from build123d import *

# Parameters (mm, degrees)
BOSS_EXTRUDE1_DEPTH = 12.7
CUT_EXTRUDE1_DEPTH  = 6.35
CUT_EXTRUDE2_DEPTH  = 233.052537155
SKETCH5_R           = 3.675
BOSS_EXTRUDE2_DEPTH = 12.7


with BuildPart() as part:
    # Sketch1 → Boss-Extrude1 (new, symmetric)
    with BuildSketch(Plane.XY):
        with BuildLine():
            Line((0, 163.1), (0, 125))
            ThreePointArc((0, 125), (88.388347648, 88.388347648), (125, 0))
            Line((125, 0), (163.1, 0))
            ThreePointArc((163.1, 0), (115.329116012, 115.329116012), (0, 163.1))
        make_face()
    extrude(amount=BOSS_EXTRUDE1_DEPTH, both=True)

    # Sketch3 → Cut-Extrude1 (cut, symmetric)
    with BuildSketch(Plane.XY):
        with BuildLine():
            Line((25.4, 161.110055552), (19.466584917, 123.474904623))
            ThreePointArc((19.466584917, 123.474904623), (88.388347648, 88.388347648), (123.474904623, 19.466584917))
            Line((123.474904623, 19.466584917), (161.110055552, 25.4))
            ThreePointArc((161.110055552, 25.4), (115.329116012, 115.329116012), (25.4, 161.110055552))
        make_face()
    extrude(amount=CUT_EXTRUDE1_DEPTH, both=True, mode=Mode.SUBTRACT)

    # Sketch4 → Cut-Extrude2 (cut, through all)
    with BuildSketch(Plane.XY.offset(12.7)):
        with BuildLine():
            ThreePointArc((18.724684767, 139.626667691), (99.614808513, 99.614808513), (139.626667691, 18.724684767))
            ThreePointArc((139.626667691, 18.724684767), (136.90184543, 15.155849254), (133.333009917, 17.880671515))
            ThreePointArc((133.333009917, 17.880671515), (95.124681201, 95.124681201), (17.880671515, 133.333009917))
            ThreePointArc((17.880671515, 133.333009917), (15.155849254, 136.90184543), (18.724684767, 139.626667691))
        make_face()
        with BuildLine():
            ThreePointArc((20.708615854, 152.170890392), (108.592878802, 108.592878802), (152.170890392, 20.708615854))
            ThreePointArc((152.170890392, 20.708615854), (149.453021799, 17.134481891), (145.878887836, 19.852350483))
            ThreePointArc((145.878887836, 19.852350483), (104.102751491, 104.102751491), (19.852350483, 145.878887836))
            ThreePointArc((19.852350483, 145.878887836), (17.134481891, 149.453021799), (20.708615854, 152.170890392))
        make_face()
    extrude(amount=-CUT_EXTRUDE2_DEPTH, mode=Mode.SUBTRACT)

    # Sketch5 → Boss-Extrude2 (add)
    with BuildSketch(Plane(origin=(0, 0, 0), x_dir=(1, 0, 0), z_dir=(0, 1, 0))):
        Polygon((163.1, -12.7), (201.2, -12.7), (201.2, 12.7), (163.1, 12.7), (163.1, 50.8), (125, 50.8), (125, 12.7), (86.9, 12.7), (86.9, -12.7), (125, -12.7), (125, -50.8), (163.1, -50.8), align=None)
        with Locations(Location((105.95, 0, 0), (0, 0, 270))):
            Circle(SKETCH5_R, mode=Mode.SUBTRACT)
        with Locations(Location((182.15, 0, 0), (0, 0, 270))):
            Circle(SKETCH5_R, mode=Mode.SUBTRACT)
        with Locations(Location((144.05, -38.1, 0), (0, 0, 270))):
            Circle(SKETCH5_R, mode=Mode.SUBTRACT)
        with Locations(Location((144.05, 38.1, 0), (0, 0, 270))):
            Circle(SKETCH5_R, mode=Mode.SUBTRACT)
    extrude(amount=BOSS_EXTRUDE2_DEPTH)


solid = part.part
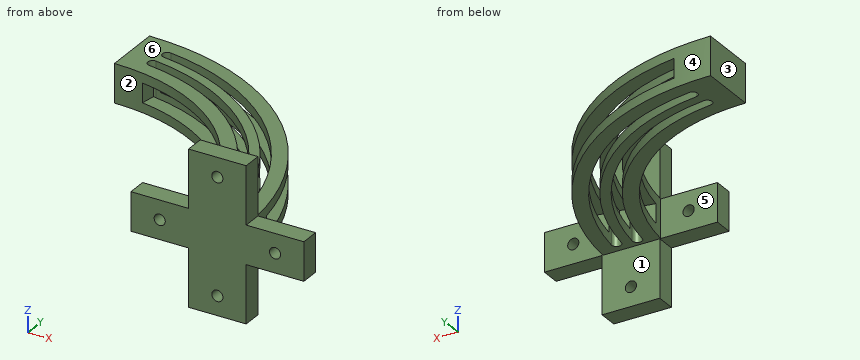
Geometry check sheet. Reference: the model listing, model coordinates, mm. Face numbers are marked on the shaded views. A direction names the side the tool comes from. Give positions to 0.01 mm unless a question says otherwise; leave off trailing zeros. Order: outer loops, then holes, each group sorted by start corner. A loop starts at its lowest first (then second) coordinate and runs counter-clockwise, first axis right, second up.
1. Sectioned sample at C-C (x = 70). Record the boundary of the cut face in (y, z), then the cut area to 3 significant figures.
Completed:
outline: (103.56, -12.7) - (114.88, -12.7) - (114.88, -6.35) - (103.56, -6.35) - close; (103.56, 6.35) - (114.88, 6.35) - (114.88, 12.7) - (103.56, 12.7) - close; (122.25, -12.7) - (129.52, -12.7) - (129.52, -6.35) - (122.25, -6.35) - close; (122.25, 6.35) - (129.52, 6.35) - (129.52, 12.7) - (122.25, 12.7) - close; (136.69, -12.7) - (147.31, -12.7) - (147.31, -6.35) - (136.69, -6.35) - close; (136.69, 6.35) - (147.31, 6.35) - (147.31, 12.7) - (136.69, 12.7) - close
area: 371 mm2
2. Sectioned sample at B-B (y = 38). Record the boundary of the cut face in (x, z), then the cut area to 3 significant figures.
Completed:
outline: (119.08, -12.7) - (129.05, -12.7) - (129.05, -6.35) - (119.08, -6.35) - close; (119.08, 6.35) - (129.05, 6.35) - (129.05, 12.7) - (119.08, 12.7) - close; (135.65, -12.7) - (142.23, -12.7) - (142.23, -6.35) - (135.65, -6.35) - close; (135.65, 6.35) - (142.23, 6.35) - (142.23, 12.7) - (135.65, 12.7) - close; (148.8, -12.7) - (158.61, -12.7) - (158.61, -6.35) - (148.8, -6.35) - close; (148.8, 6.35) - (158.61, 6.35) - (158.61, 12.7) - (148.8, 12.7) - close
area: 335 mm2
3. Scan lines: line 1 (Z direction, x = 144, y = 10); line 2 (X direction, y = 3, z = -38); line 3 (X direction, y = 50, z = 11.5). Record each from-to range of solid material in increasing order.
Completed:
line 1: z = -50.8 to -41.77, -34.43 to 34.43, 41.77 to 50.8
line 2: x = 125 to 140.38, 147.72 to 163.1
line 3: x = 114.56 to 124.89, 131.71 to 138.47, 145.21 to 155.25
4. Access from +Z, -Z, +X, -X, +Y, -Y to the whole of each face (thin tool, end or side, straight path). Record for the marked faces 1, 2 and 3.
Completed:
face 1: +X, +Y
face 2: +Z, -Z, -X
face 3: +Z, -Z, -X, +Y, -Y
5. Sectioned sample at A-A (z = 38.1). Record the boundary of the cut face in (x, y) (3 decimals).
Completed:
outline: (125, 0) - (140.375, 0) - (140.375, 12.7) - (125, 12.7) - close; (147.725, 0) - (163.1, 0) - (163.1, 12.7) - (147.725, 12.7) - close
6. Draft check along Y on the marked faces 4, 5 and 6. Enter one of: pulls with the +Y half, pulls with the -Y half, needs draft (parallel to the pull), parting line crosses it, or undercut.
Completed:
face 4: pulls with the +Y half
face 5: undercut
face 6: needs draft
7. Sectioned sample at D-D (y = 136). Record the boundary of the cut face in (x, z).
Completed:
outline: (0, -12.7) - (15.16, -12.7) - (15.16, 12.7) - (0, 12.7) - close; (36.75, -12.7) - (56.38, -12.7) - (56.38, -6.35) - (36.75, -6.35) - close; (36.75, 6.35) - (56.38, 6.35) - (56.38, 12.7) - (36.75, 12.7) - close; (71.34, -12.7) - (90.03, -12.7) - (90.03, -6.35) - (71.34, -6.35) - close; (71.34, 6.35) - (90.03, 6.35) - (90.03, 12.7) - (71.34, 12.7) - close
8. Depth check by flat-ended pin: pin 1 (4 mm diameter, centred on y = 8, z = 3.5, fed in from -X); pin 2 (14 mm diameter, centred on y = 5, z = -35.5, fed in from -X); pin 3 (14 mm diameter, centred on x = 186, y = 5.5, fed in from +Z). Enter the tip coordinate at first touch or a pass-through.
Completed:
pin 1: stops at x = 86.9
pin 2: stops at x = 125
pin 3: stops at z = 12.7
